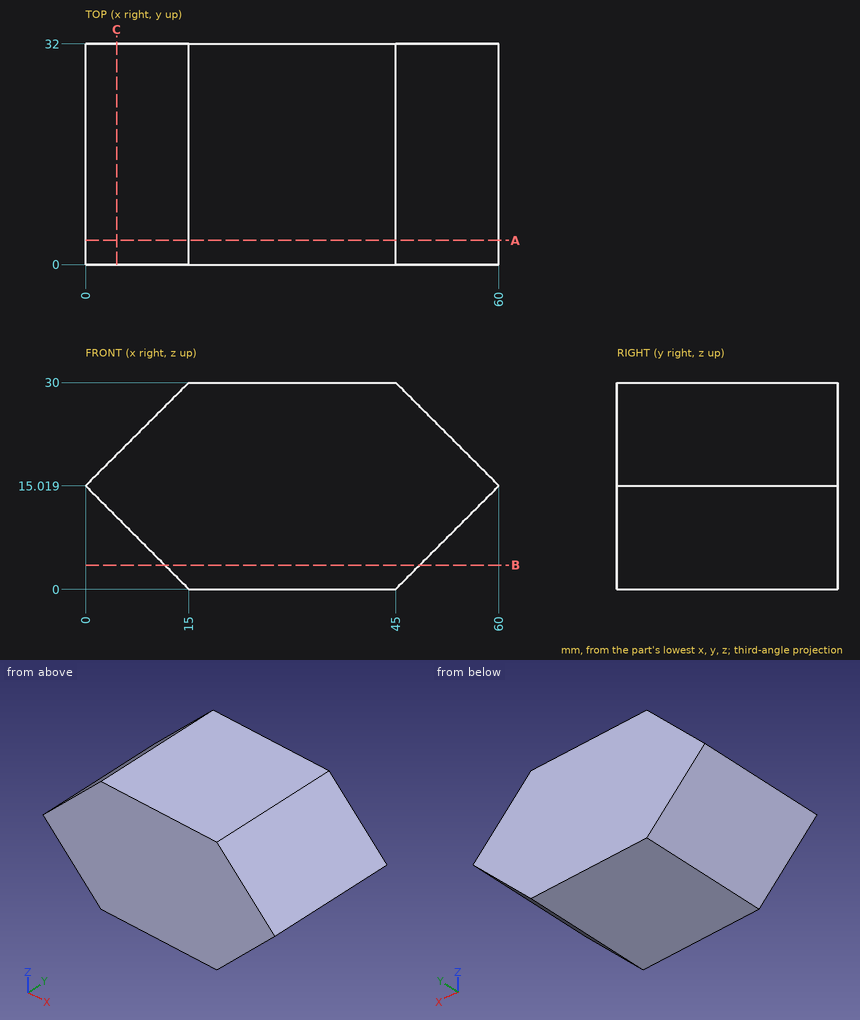
Here's the drawing with two shaded views (mm, measured from the low corner). I have some questions. Round coordinates to 2 decimals unless told otherwise and drop trailing zeros. Loops run counter-clockwise (first coordinate to the right, second up) from the corner with the lowest first, then second, coordinate; pieces in that order, holes last. Notation, with made-up numbers: M -20,36.25 L 16,36.25 A24 ccw 16,50.25 Z; hole C 49,74 d5. An arc over 180 degrees is marked long. Put each result on its own line as item: value.
Q1. Imagine slicing it at A-A (y = 3.5). Write out the boundary of the cut face in (x, z), then the cut area to 3 significant figures.
Check result:
outline: M 0,15.02 L 15,0 L 45,0 L 60,15.02 L 45,30 L 15,30 Z
area: 1,350 mm2
Q2. Imagine slicing it at B-B (z = 3.5). Write out the boundary of the cut face in (x, y).
Check result:
outline: M 11.5,0 L 48.5,0 L 48.5,32 L 11.5,32 Z
Q3. Imagine slicing it at C-C (x = 4.5). Write out the boundary of the cut face in (y, z), then the cut area to 3 significant figures.
Check result:
outline: M 0,10.51 L 32,10.51 L 32,19.51 L 0,19.51 Z
area: 288 mm2
Q4. For pin 1 (1.5 mm diameter, centred on x = 13.5, y = 13, fed in from +Z); pin 2 (12 mm diameter, centred on y = 4.5, z = 4, fed in from -X); pin 3 (1 mm diameter, centred on y = 24, z = 22.5, fed in from +X), each with a flat end and sliding along its axis, tell me the tip position at first contact or that it passes through.
Check result:
pin 1: z = 29.25
pin 2: x = 5.01
pin 3: x = 53.01
Q5. I need wall thicknesses on probe 1 along X at (y, z) = (23.5, 1.5); probe 2 along Z at (x, y) = (8, 27.5); probe 3 along Z at (x, y) = (50, 19) (1 decimal). Which ranges of each line are inside material? Lowest first, please.
Check result:
probe 1: 13.5 to 46.5
probe 2: 7.01 to 23.01
probe 3: 5 to 25
